from build123d import *

# Parameters (mm, degrees)
SKETCH1_W           = 40
SKETCH1_H           = 40
BOSS_EXTRUDE1_DEPTH = 6
SKETCH3_R           = 6
CUT_EXTRUDE1_DEPTH  = 29.956627751


with BuildPart() as part:
    # Sketch1 → Boss-Extrude1 (new body)
    with BuildSketch(Plane.XY):
        with Locations((-0.03035818, 0.031750845)):
            Rectangle(SKETCH1_W, SKETCH1_H)
    extrude(amount=BOSS_EXTRUDE1_DEPTH)

    # Sketch3 → Cut-Extrude1 (cut, through all)
    with BuildSketch(Plane.XY):
        with Locations((0.03811678, -6.611407744)):
            Circle(SKETCH3_R)
        with BuildLine():
            ThreePointArc((-1.563550895, 15.055123875), (-7.521124365, 15.038743131), (-11.132245635, 10.300309513))
            ThreePointArc((-11.132245635, 10.300309513), (-9.975977933, 8.583173649), (-8.258842069, 9.739441351))
            ThreePointArc((-8.258842069, 9.739441351), (-6.218325676, 12.416961919), (-2.851912471, 12.426218095))
            ThreePointArc((-2.851912471, 12.426218095), (-0.893278793, 13.096490197), (-1.563550895, 15.055123875))
        make_face()
        with BuildLine():
            ThreePointArc((10.897165218, 10.597004263), (7.169871935, 15.244609534), (1.213718069, 15.113532793))
            ThreePointArc((1.213718069, 15.113532793), (0.592128311, 13.138909601), (2.566751502, 12.517319844))
            ThreePointArc((2.566751502, 12.517319844), (5.932362539, 12.591386656), (8.038523611, 9.965189961))
            ThreePointArc((8.038523611, 9.965189961), (9.783751566, 8.851776308), (10.897165218, 10.597004263))
        make_face()
        with BuildLine():
            ThreePointArc((15.180796373, -1.924768002), (16.490511142, 3.887081721), (12.674430025, 8.462065316))
            ThreePointArc((12.674430025, 8.462065316), (10.743052573, 7.716886336), (11.488231553, 5.785508884))
            ThreePointArc((11.488231553, 5.785508884), (13.644563477, 3.20034812), (12.904490171, -0.083721771))
            ThreePointArc((12.904490171, -0.083721771), (13.122120157, -2.142397987), (15.180796373, -1.924768002))
        make_face()
        with BuildLine():
            ThreePointArc((8.06168094, -13.081043006), (13.422161827, -10.481390213), (14.619740374, -4.645402241))
            ThreePointArc((14.619740374, -4.645402241), (12.832941842, -3.60000204), (11.78754164, -5.386800572))
            ThreePointArc((11.78754164, -5.386800572), (11.110832531, -8.684510129), (8.081815142, -10.153481604))
            ThreePointArc((8.081815142, -10.153481604), (6.60796734, -11.607195205), (8.06168094, -13.081043006))
        make_face()
        with BuildLine():
            ThreePointArc((-5.099341956, -14.470918126), (0.275353607, -17.041053839), (5.584790746, -14.338679466))
            ThreePointArc((5.584790746, -14.338679466), (5.288066872, -12.289907756), (3.239295163, -12.586631629))
            ThreePointArc((3.239295163, -12.586631629), (0.239120783, -14.113647422), (-2.797928816, -12.661355))
            ThreePointArc((-2.797928816, -12.661355), (-4.853416949, -12.415429993), (-5.099341956, -14.470918126))
        make_face()
        with BuildLine():
            ThreePointArc((-14.391753639, -5.047789047), (-13.050098782, -10.852348653), (-7.62691751, -13.3185309))
            ThreePointArc((-7.62691751, -13.3185309), (-6.210127596, -11.809154567), (-7.719503929, -10.392364653))
            ThreePointArc((-7.719503929, -10.392364653), (-10.783951079, -8.998812644), (-11.542072595, -5.718862139))
            ThreePointArc((-11.542072595, -5.718862139), (-12.63137657, -3.958485071), (-14.391753639, -5.047789047))
        make_face()
        with BuildLine():
            ThreePointArc((-12.81817858, 8.092535837), (-16.519857902, 3.424504113), (-15.066698607, -2.353149221))
            ThreePointArc((-15.066698607, -2.353149221), (-13.003266608, -2.519759429), (-12.8366564, -0.456327431))
            ThreePointArc((-12.8366564, -0.456327431), (-13.657785113, 2.808419294), (-11.566097582, 5.446158252))
            ThreePointArc((-11.566097582, 5.446158252), (-10.868949288, 7.395387544), (-12.81817858, 8.092535837))
        make_face()
    extrude(amount=CUT_EXTRUDE1_DEPTH, mode=Mode.SUBTRACT)


solid = part.part
Geometry check sheet. Reference: the model listing, model coordinates, mm. A direction names the side the tool comes from. Round coordinates to 2 decimals unless told otherwise and drop trailing zeros. Write each loop counter-clockwise with the first axis right and the second up, starting at its lowest first coordinate (ties: lowest second). Pieces come first, ordered by that corner, then holes. Notation, with made-up numbers: (0, 10) - (40, 10) arc R25 cw to (40, 41) - close; hole circle Ø9 at (66.5, -6.5). An arc over 180 degrees is marked (long way). One line per item, written item: value.
1. Cross-section at C-C on x = -7. Record the boundary of the cut face in (y, z), and give its area (3 significant figures).
The answers:
outline: (-19.97, 0) - (-13.16, 0) - (-13.16, 6) - (-19.97, 6) - close; (-10.56, 0) - (11.9, 0) - (11.9, 6) - (-10.56, 6) - close; (15.27, 0) - (20.03, 0) - (20.03, 6) - (15.27, 6) - close
area: 204 mm^2
2. Mould release check, pull along X, two halves, no side actions. Record for faces 1 (the face through (-10.01, 8.59, 2.96)), 2 (the face through (0, 20.032, 3)): released by +X, released by -X, zero draft, split by the parting line, or undercut.
The answers:
face 1: undercut
face 2: zero draft
3. Set-up check for faces 3 (the face through (0, 0, 0)), 4 (the face through (7.248, 15.208, 2.958)): record each of +Z, -Z, +X, -X, +Y, -Y from which the full face is reachable in a straight line by a thin tool's end or side.
The answers:
face 3: -Z, +X, -X, +Y, -Y
face 4: +Z, -Z
4. Cross-section at D-D on y = -11. Record the boundary of the cut face in (x, z), and give its area (3 significant figures).
The answers:
outline: (-20.03, 0) - (-12.93, 0) - (-12.93, 6) - (-20.03, 6) - close; (-6.49, 0) - (-4.05, 0) - (-4.05, 6) - (-6.49, 6) - close; (4.13, 0) - (6.74, 0) - (6.74, 6) - (4.13, 6) - close; (12.97, 0) - (19.97, 0) - (19.97, 6) - (12.97, 6) - close
area: 115 mm^2
5. Cross-section at B-B on z = 2. Give the number of separate pieces and of enclosed holes in the cut face, and give its area (3 significant figures).
The answers:
separate pieces: 1
enclosed holes: 8
area: 1,240 mm^2
6. Cross-section at A-A on y = 1.5. Record the boundary of the cut face in (x, z), and give its area (3 significant figures).
The answers:
outline: (-20.03, 0) - (-16.65, 0) - (-16.65, 6) - (-20.03, 6) - close; (-13.71, 0) - (13.66, 0) - (13.66, 6) - (-13.71, 6) - close; (16.63, 0) - (19.97, 0) - (19.97, 6) - (16.63, 6) - close
area: 205 mm^2
7. Scan lines: L1, parallel to Y at x = 0, z = 0.8; L2, parallel to X at y = -6.5, z = 5.25; L3, parallel to X at y = -7.5, z = 2.45. Record each from-to range of solid material in increasing order.
The answers:
L1: y = -19.97 to -17.04, -14.11 to -12.61, -0.61 to 20.03
L2: x = -20.03 to -14.57, -11.64 to -5.96, 6.04 to 11.91, 14.84 to 19.97
L3: x = -20.03 to -14.51, -11.53 to -5.9, 5.97 to 11.73, 14.74 to 19.97
8. Depth check by flat-ended pin: pin 1 Ø9.5 at (x, y) = (0.04, -6.61) entering from +Z; pin 2 Ø6 at (x, y) = (-1, 6.5) entering from -Z. Enter the tip coordinate at first touch or a pass-through.
The answers:
pin 1: passes through
pin 2: stops at z = 0
